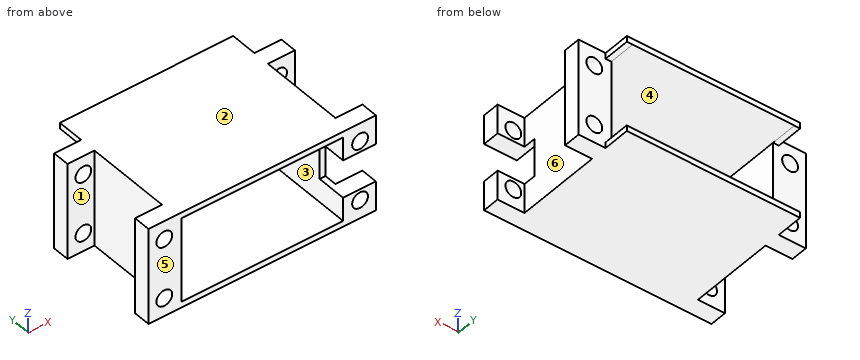
```python
from build123d import *

# Parameters (mm, degrees)
SKETCH1_W               = 45
SKETCH1_H               = 25
SKETCH1_W_2             = 42
SKETCH1_H_2             = 22
BOSS_EXTRUDE1_DEPTH     = 38
CUT_EXTRUDE2_START      = -46
SKETCH3_W               = 21.995206391
SKETCH3_H               = 7
CUT_EXTRUDE2_DEPTH      = 47
SKETCH4_W               = 25
SKETCH4_H               = 4.4
BOSS_EXTRUDE3_DEPTH     = 7
SKETCH8_R               = 2.05
CUT_EXTRUDE5_DEPTH      = 4.4
SKETCH6_W               = 9.8
SKETCH6_H               = 10.757060019
CUT_EXTRUDE4_DEPTH      = 8
CUT_EXTRUDE4_DEPTH_BACK = 7
MIRROR2_START           = -46
MIRROR2_COPY_1_SKETCH_W = 21.995206391
MIRROR2_COPY_1_SKETCH_H = 7
MIRROR2_COPY_1_DEPTH    = 47
MIRROR2_COPY_2_SKETCH_W = 25
MIRROR2_COPY_2_SKETCH_H = 4.4
MIRROR2_COPY_2_DEPTH    = 7
MIRROR2_COPY_3_SKETCH_R = 2.05
MIRROR2_COPY_3_DEPTH    = 4.4
SKETCH6_2_W             = 9.8
SKETCH6_2_H             = 10.757060019
CUT_EXTRUDE6_DEPTH      = 15


with BuildPart() as part:
    # Sketch1 → Boss-Extrude1 (new body)
    with BuildSketch(Plane(origin=(0, 0, 0), x_dir=(1, 0, 0), z_dir=(0, 1, 0))):
        with Locations((21, 11)):
            Rectangle(SKETCH1_W, SKETCH1_H)
        with Locations((21, 11)):
            Rectangle(SKETCH1_W_2, SKETCH1_H_2, mode=Mode.SUBTRACT)
    extrude(amount=BOSS_EXTRUDE1_DEPTH)

    # Sketch3 → Cut-Extrude2 (cut)
    with BuildSketch(Plane(origin=(43.5, 0, 0), x_dir=(0, 0, -1), z_dir=(1, 0, 0)).offset(CUT_EXTRUDE2_START)):
        with Locations((11.002396805, 34.5)):
            Rectangle(SKETCH3_W, SKETCH3_H)
    cut_extrude2 = extrude(amount=CUT_EXTRUDE2_DEPTH, mode=Mode.SUBTRACT)

    # Sketch4 → Boss-Extrude3 (add)
    with BuildSketch(Plane(origin=(43.5, 0, 0), x_dir=(0, 0, -1), z_dir=(1, 0, 0))):
        with Locations((11, 28.8)):
            Rectangle(SKETCH4_W, SKETCH4_H)
    boss_extrude3 = extrude(amount=BOSS_EXTRUDE3_DEPTH)

    # Sketch8 → Cut-Extrude5 (cut)
    with BuildSketch(Plane(origin=(0, 31, 0), x_dir=(1, 0, 0), z_dir=(0, 1, 0))):
        with Locations((46.4, 18.75)):
            Circle(SKETCH8_R)
        with Locations((46.399285585, 3.250377991)):
            Circle(SKETCH8_R)
    cut_extrude5 = extrude(amount=-CUT_EXTRUDE5_DEPTH, mode=Mode.SUBTRACT)

    # Mirror1: Cut-Extrude2, Boss-Extrude3, Cut-Extrude5 across plane
    add(cut_extrude2.mirror(Plane(origin=(21, 0, 0), x_dir=(0, 0, 1), z_dir=(1, 0, 0))), mode=Mode.SUBTRACT)
    add(boss_extrude3.mirror(Plane(origin=(21, 0, 0), x_dir=(0, 0, 1), z_dir=(1, 0, 0))))
    add(cut_extrude5.mirror(Plane(origin=(21, 0, 0), x_dir=(0, 0, 1), z_dir=(1, 0, 0))), mode=Mode.SUBTRACT)

    # Sketch6 → Cut-Extrude4 (cut, two sides)
    with BuildSketch(Plane(origin=(43.5, 0, 0), x_dir=(0, 0, -1), z_dir=(1, 0, 0))) as cut_extrude4_sk:
        with Locations((11, 2.32146999)):
            Rectangle(SKETCH6_W, SKETCH6_H)
    extrude(amount=CUT_EXTRUDE4_DEPTH, mode=Mode.SUBTRACT)
    extrude(cut_extrude4_sk.sketch, amount=-CUT_EXTRUDE4_DEPTH_BACK, mode=Mode.SUBTRACT)

    # Mirror2: Cut-Extrude2, Boss-Extrude3, Cut-Extrude5 across plane
    add(cut_extrude2.mirror(Plane.ZX.offset(15.5)), mode=Mode.SUBTRACT)
    add(boss_extrude3.mirror(Plane.ZX.offset(15.5)))
    add(cut_extrude5.mirror(Plane.ZX.offset(15.5)), mode=Mode.SUBTRACT)

    # Mirror2 copy 1 sketch → Mirror2 copy 1 (cut)
    with BuildSketch(Plane(origin=(-1.5, 31, 0), x_dir=(0, 0, -1), z_dir=(-1, 0, 0)).offset(MIRROR2_START)):
        with Locations((11.002396805, 34.5)):
            Rectangle(MIRROR2_COPY_1_SKETCH_W, MIRROR2_COPY_1_SKETCH_H)
    extrude(amount=MIRROR2_COPY_1_DEPTH, mode=Mode.SUBTRACT)

    # Mirror2 copy 2 sketch → Mirror2 copy 2 (add)
    with BuildSketch(Plane(origin=(-1.5, 31, 0), x_dir=(0, 0, -1), z_dir=(-1, 0, 0))):
        with Locations((11, 28.8)):
            Rectangle(MIRROR2_COPY_2_SKETCH_W, MIRROR2_COPY_2_SKETCH_H)
    extrude(amount=MIRROR2_COPY_2_DEPTH)

    # Mirror2 copy 3 sketch → Mirror2 copy 3 (cut)
    with BuildSketch(Plane(origin=(42, 0, 0), x_dir=(-1, 0, 0), z_dir=(0, -1, 0))):
        with Locations((46.4, 18.75)):
            Circle(MIRROR2_COPY_3_SKETCH_R)
        with Locations((46.399285585, 3.250377991)):
            Circle(MIRROR2_COPY_3_SKETCH_R)
    extrude(amount=-MIRROR2_COPY_3_DEPTH, mode=Mode.SUBTRACT)

    # Sketch6<2> → Cut-Extrude6 (cut)
    with BuildSketch(Plane(origin=(43.5, 0, 0), x_dir=(0, 0, -1), z_dir=(1, 0, 0))):
        with Locations((11, 2.32146999)):
            Rectangle(SKETCH6_2_W, SKETCH6_2_H)
    extrude(amount=CUT_EXTRUDE6_DEPTH, mode=Mode.SUBTRACT)


solid = part.part
```
Can you work these out from the model? Positions are in its coordinate system, mm. Face numbers are marked on the shaded views. A direction names the side the tool comes from. Give positions to 0.01 mm unless a question says otherwise; leave off trailing zeros. Loops run counter-clockwise (first coordinate to the right, second up) from the corner with the lowest first, then second, coordinate; pieces in that order, holes last. Notation, with made-up numbers: M 84,26 L 103,26 A35 cw 103,59 Z; hole C -28.75,79 d5. An arc over 180 degrees is marked long. One line per item, written item: value.
(1) We'd pull the mould along Y, two halves only. Please class the marked faces 4, 5 and 6: released by +Y, released by -Y, zero draft, split by the parting line, or undercut.
Returned:
face 4: zero draft
face 5: released by -Y
face 6: undercut
(2) Suppose I cut it at A-A on x = -4.4. List the corners of the cut face in (y, z) for me.
Returned:
outline: M 0,-23.5 L 4.4,-23.5 L 4.4,-20.8 L 0,-20.8 Z; M 0,-16.7 L 4.4,-16.7 L 4.4,-5.3 L 0,-5.3 Z; M 0,-1.2 L 4.4,-1.2 L 4.4,1.5 L 0,1.5 Z; M 26.6,-23.5 L 31,-23.5 L 31,-20.8 L 26.6,-20.8 Z; M 26.6,-16.7 L 31,-16.7 L 31,-5.3 L 26.6,-5.3 Z; M 26.6,-1.2 L 31,-1.2 L 31,1.5 L 26.6,1.5 Z
(3) Suppose I cut it at C-C on z = -18.75. Count the separate pieces of the cut face and the enclosed holes in it, plus the area to 3 significant figures.
Returned:
separate pieces: 6
enclosed holes: 0
area: 144 mm^2
(4) Which directions (+Z, -Z, +X, -X, +Y, -Y) give clear straight access to the entire face, cutting with the end or side of a thin tool? Please do the marked faces 1, 2 and 3.
Returned:
face 1: +Z, -Z, -X
face 2: +Z, +X, -X, +Y, -Y
face 3: +Y, -Y
(5) Suppose I cut it at B-B on z = -15. List the corners of the cut face in (x, y) for me, plus the area to 3 significant figures.
Returned:
outline: M -8.5,0 L 0,0 L 0,31 L -8.5,31 L -8.5,26.6 L -1.5,26.6 L -1.5,4.4 L -8.5,4.4 Z; M 42,7.7 L 43.5,7.7 L 43.5,26.6 L 50.5,26.6 L 50.5,31 L 42,31 Z
area: 174 mm^2
(6) Will these pins go through, and if not, where does the flat tip stop? pin 1 (8 mm diameter, centred on y = 13.5, z = -6.5, fed in from -X); pin 2 (2 mm diameter, centred on x = -5, z = -15.5, fed in from +Y).
Returned:
pin 1: x = -1.5
pin 2: y = 31
(7) I need wall thicknesses on line 1 (X direction, y = 27.75, z = -18.75); line 2 (Z direction, x = 46.4, y = 2.8); line 3 (X direction, y = 9.5, z = -6.75). Which ranges of each line are inside material? Lowest first, please.
Returned:
line 1: -8.5 to -6.45, -2.35 to 0, 42 to 44.35, 48.45 to 50.5
line 2: -23.5 to -20.8, -16.7 to -15.9, -6.1 to -5.3, -1.2 to 1.5
line 3: -1.5 to 0, 42 to 43.5
(8) Suppose I cut it at D-D on x = 35. List the corners of the cut face in (y, z) for me, plus the area to 3 significant figures.
Returned:
outline: M 0,-23.5 L 38,-23.5 L 38,-22 L 0,-22 Z; M 0,0 L 38,0 L 38,1.5 L 0,1.5 Z
area: 114 mm^2
